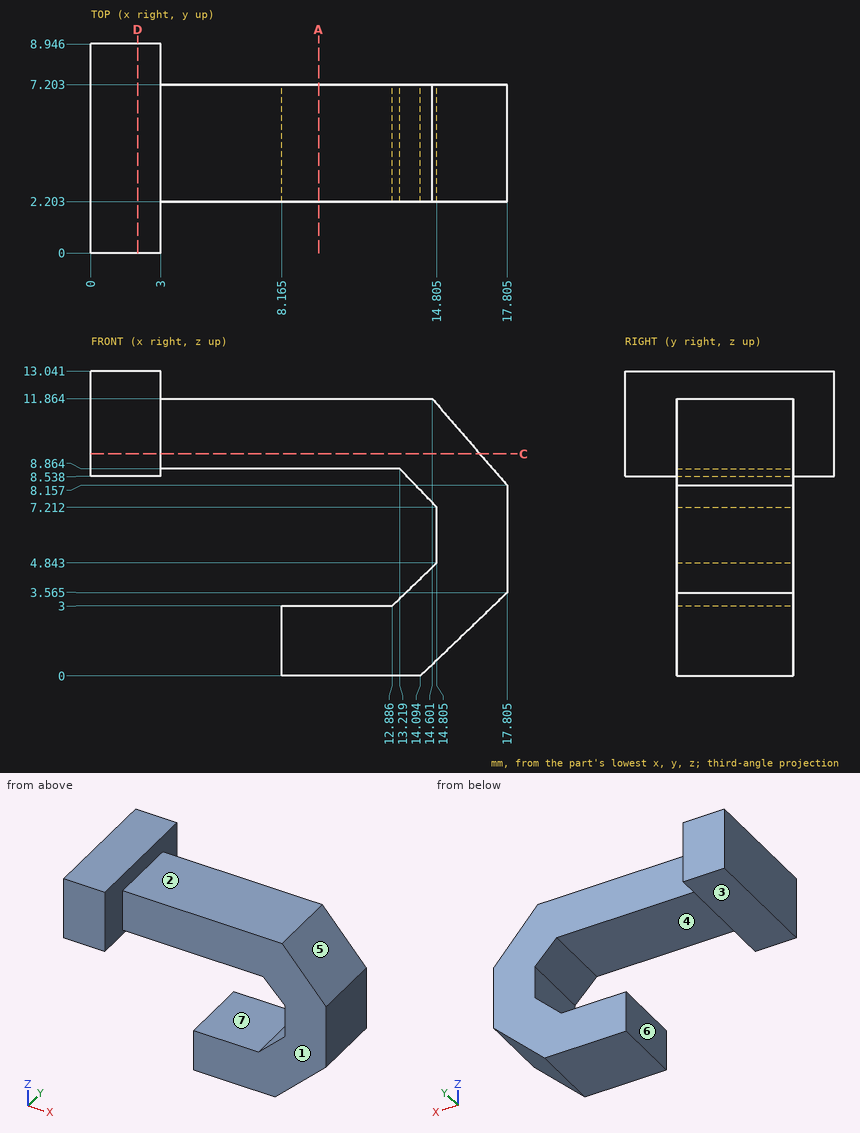
Geometry check sheet. Reference: drawing and pictorial views, mm from the part's lowest x, y, z. A direction names the side the tool comes from. Give positions to 0.01 mm unless a question says otherwise; leave off trailing zeros. Order: outer loops, then holes, each group sorted by start corner. A loop starts at its lowest first (then second) coordinate and runs counter-clockwise, first axis right, second up. Notation, with made-up numbers: M 2,42 L 30,42 A25 cw 30,81 Z; hole C 30,21.25 d9. An arc over 180 degrees is marked long. Return JSON: item names as keys, results as strings. Group by question number.
1) Scan lines: line 1 (Z direction, x = 8.5, y = 4.5) (1 decimal); line 2 (X direction, y = 3.5, z = 12.75); line 3 (Y direction, x = 6, z = 9.75). Record each from-to range of solid material in increasing order.
2) Mould release check, pull along Z, two halves, no side actions. Record for the marked faces 5, 6 and 7: pulls with the +Z half, pulls with the -Z half, needs draft (parallel to the pull), parting line crosses it, or undercut.
3) Section check D-D on x = 2. Record the cut outline in (y, z).
4) Section check C-C on z = 9.5. Record the cut outline in (x, y) (1 decimal).
5) Go/stop test with flat-tipped pins: pin 1 Ø1 at (x, y) = (11.5, 6) entering from +Z; pin 2 Ø0.7 at (y, z) = (4.5, 6.5) entering from -X (1 decimal); pin 3 Ø2.5 at (x, y) = (1, 6.5) entering from -Z; pin 4 Ø2 at (x, z) = (5.5, 7) entering from -Y. Record where each tip stops, or that it passes through.
6) Section check A-A on x = 9.75. Record the cut outline in (y, z) (1 decimal).
7) Access from +Z, -Z, +X, -X, +Y, -Y to the whole of each face (thin tool, end or side, straight path). Record for the marked faces 1, 2, 3 and 4.
Answer block:
{
 "1": {"line 1": "z = 0 to 3, 8.9 to 11.9", "line 2": "x = 0 to 3", "line 3": "y = 2.2 to 7.2"},
 "2": {"face 5": "pulls with the +Z half", "face 6": "needs draft", "face 7": "undercut"},
 "3": {"outline": "M 0,8.54 L 8.95,8.54 L 8.95,13.04 L 0,13.04 Z"},
 "4": {"outline": "M 0,0 L 3,0 L 3,2.2 L 16.6,2.2 L 16.6,7.2 L 3,7.2 L 3,8.9 L 0,8.9 Z"},
 "5": {"pin 1": "stops at z = 11.86", "pin 2": "stops at x = 14.8", "pin 3": "stops at z = 8.54", "pin 4": "passes through"},
 "6": {"outline": "M 2.2,0 L 7.2,0 L 7.2,3 L 2.2,3 Z; M 2.2,8.9 L 7.2,8.9 L 7.2,11.9 L 2.2,11.9 Z"},
 "7": {"face 1": "+Z, -Z, +X, -Y", "face 2": "+Z, +X, +Y, -Y", "face 3": "-Z, -X, +Y, -Y", "face 4": "+Y, -Y"}
}
